For this review, take the finished solid that the model builds, in its own axes (mm). A direction names the side the tool comes from. Give positions to 0.01 mm unless a question says otherwise; leave off trailing zeros. Write each loop counter-clockwise with the first axis right and the second up, starting at its lowest first coordinate (ties: lowest second). Pieces come first, ordered by that corner, then holes.
from build123d import *

# Parameters (mm, degrees)
F0_W     = 38.1
F0_H     = 10
F1_DEPTH = 63.5
F2_W     = 38.0510927618
F2_H     = 7.2934785858
F3_DEPTH = 38.1
F4_W     = 38.0510927618
F4_H     = 15
F5_DEPTH = 76.2


with BuildPart() as f1:
    # F0 (on Front) → F1 (new body)
    with BuildSketch(Plane.XZ):
        Rectangle(F0_W, F0_H)
    extrude(amount=-F1_DEPTH)

    # F2 (on face) → F3 (join)
    with BuildSketch(Plane.XY.offset(5)):
        with Locations((-0.0244536191, -3.6467392929)):
            Rectangle(F2_W, F2_H)
    extrude(amount=-F3_DEPTH)

    # F4 (on face) → F5 (join)
    with BuildSketch(Plane.XZ.offset(7.2934785858)):
        with Locations((-0.0244536191, -2.5)):
            Rectangle(F4_W, F4_H)
    extrude(amount=F5_DEPTH)


solid = f1.part
(1) We need section B-B (z = -14). Write out the cut boundary in (x, y), and give its area (3 significant figures).
(2) Clearance check with flat-ended pins moving along their axes: pin 1 Ø1 at (y, z) = (-42, -2) entering from +X; pin 2 Ø8.5 at (x, z) = (0, -22.5) entering from +Y; pin 3 Ø2 at (x, y) = (14, -24.5) entering from -Z. State where each tip first meets the part, or that it passes through.
(3) Tool access review of faces 1 (the flat face through (0, 0, -19)), 2 (the flat face through (0, -45, -10)), 3 (the flat face through (-19.05, -15, -3)): name each direction out of +Z, -Z, +X, -X, +Y, -Y from which nothing blocks a thin tool from reaching the whole face with its end or side.
(4) We need section C-C (y = 30). Write out the cut boundary in (x, z).
(5) For L1, parallel to Z at x = -3, y = 34.5; L2, parallel to Y at x = 15, z = -20.5; L3, parallel to Z at x = 4.5, y = -42, list the stretches that pass through material, from the lowest coordinate up.
(6) We need section A-A (x = 2). Write out the cut boundary in (y, z), and give its area (3 significant figures).
The answers:
1. outline: (-19.05, -7.29) - (19, -7.29) - (19, 0) - (-19.05, 0) - close
1. area: 278 mm2
2. pin 1: stops at x = 19
2. pin 2: stops at y = 0
2. pin 3: stops at z = -10
3. face 1: -Z, +X, -X, +Y
3. face 2: -Z, +X, -X, -Y
3. face 3: +Z, -Z, -X, +Y, -Y
4. outline: (-19.05, -5) - (19.05, -5) - (19.05, 5) - (-19.05, 5) - close
5. L1: z = -5 to 5
5. L2: y = -7.29 to 0
5. L3: z = -10 to 5
6. outline: (-83.49, -10) - (-7.29, -10) - (-7.29, -33.1) - (0, -33.1) - (0, -5) - (63.5, -5) - (63.5, 5) - (-83.49, 5) - close
6. area: 2,060 mm2
